Here's how the part is built. I have some questions about the finished solid (model axes, mm). Face numbers are marked on the shaded views. A direction names the side the tool comes from. Give positions to 0.01 mm unless a question says otherwise; leave off trailing zeros. Write each loop counter-clockwise with the first axis right and the second up, starting at its lowest first coordinate (ties: lowest second). Pieces come first, ordered by that corner, then holes. Notation, with made-up numbers: (54, 64.5) -> (103, 64.5) arc R28 ccw to (103, 83.5) -> close; hole circle Ø7 at (73, 81.25). An arc over 180 degrees is marked (long way). Return JSON: item names as keys, results as strings.
from build123d import *

# Parameters (mm, degrees)
F0_R     = 2.5
F0_W     = 19
F0_H     = 3
F0_W_2   = 13
F0_W_3   = 9.5
F0_R_2   = 1.25
F1_DEPTH = 2.5
F2_DEPTH = 15
F3_DEPTH = 6.5
F4_DEPTH = 2.5
F5_DEPTH = 5


# Not quite as in the source:
# - a feature names something its author has since deleted; it is built from what else it names


with BuildPart() as f1:
    # F0 (on Top) → F1 (new body)
    with BuildSketch(Plane.XY):
        Polygon((27.0149873525, -30.0875452161), (27.0149873525, 34.3124547839), (21.4149873525, 39.9124547839), (-12.9189450768, 39.9124547839), (-15.2438546447, 37.5875452161), (-27.5850126475, 37.5875452161), (-27.5850126475, -30.0875452161), (-17.9850126475, -30.0875452161), (-4.9850126475, -30.0875452161), (14.0149873525, -30.0875452161), (23.5149873525, -30.0875452161), align=None)
        with Locations((-24.5850126475, -15.0875452161)):
            Circle(F0_R, mode=Mode.SUBTRACT)
        with Locations((24.0149873525, -16.0875452161)):
            Circle(F0_R, mode=Mode.SUBTRACT)
        with Locations((-8.6850126475, 33.8492766023)):
            Circle(F0_R, mode=Mode.SUBTRACT)
        with Locations((19.3149873525, 33.8492766023)):
            Circle(F0_R, mode=Mode.SUBTRACT)
        Polygon((21.4149873525, 39.9124547839), (27.0149873525, 34.3124547839), (27.0149873525, -30.0875452161), (29.5149873525, -30.0875452161), (29.5149873525, 34.3124547839), (21.5734839439, 42.4124547839), (-13.0739709929, 42.4124547839), (-15.4701419023, 40.0875452161), (-30.0850126475, 40.0875452161), (-30.0850126475, 10), (-30.0850126475, 5), (-30.0850126475, 0), (-30.0850126475, -5), (-30.0850126475, -30.0875452161), (-27.5850126475, -30.0875452161), (-27.5850126475, 37.5875452161), (-15.2438546447, 37.5875452161), (-12.9189450768, 39.9124547839), align=None)
        with Locations((4.5149873525, -31.5875452161)):
            Rectangle(F0_W, F0_H)
        with Locations((-11.4850126475, -31.5875452161)):
            Rectangle(F0_W_2, F0_H)
        Polygon((-17.9850126475, -33.0875452161), (-17.9850126475, -30.0875452161), (-27.5850126475, -30.0875452161), (-30.0850126475, -30.0875452161), (-30.0850126475, -33.0875452161), align=None)
        with Locations((18.7649873525, -31.5875452161)):
            Rectangle(F0_W_3, F0_H)
        with Locations((19.3149873525, 33.8492766023)):
            Circle(F0_R)
        with Locations((19.3149873525, 33.8492766023)):
            Circle(F0_R_2, mode=Mode.SUBTRACT)
        with Locations((-24.5850126475, -15.0875452161)):
            Circle(F0_R)
        with Locations((-24.5850126475, -15.0875452161)):
            Circle(F0_R_2, mode=Mode.SUBTRACT)
        with Locations((24.0149873525, -16.0875452161)):
            Circle(F0_R)
        with Locations((24.0149873525, -16.0875452161)):
            Circle(F0_R_2, mode=Mode.SUBTRACT)
        with Locations((-8.6850126475, 33.8492766023)):
            Circle(F0_R)
        with Locations((-8.6850126475, 33.8492766023)):
            Circle(F0_R_2, mode=Mode.SUBTRACT)
        Polygon((29.5149873525, -30.0875452161), (27.0149873525, -30.0875452161), (23.5149873525, -30.0875452161), (23.5149873525, -33.0875452161), (29.5149873525, -33.0875452161), align=None)
        with Locations((-24.5850126475, -15.0875452161)):
            Circle(F0_R_2)
        with Locations((24.0149873525, -16.0875452161)):
            Circle(F0_R_2)
        with Locations((-8.6850126475, 33.8492766023)):
            Circle(F0_R_2)
        with Locations((19.3149873525, 33.8492766023)):
            Circle(F0_R_2)
    extrude(amount=-F1_DEPTH)

    # F0 (on Top) → F2 (join)
    with BuildSketch(Plane.XY):
        Polygon((21.4149873525, 39.9124547839), (27.0149873525, 34.3124547839), (27.0149873525, -30.0875452161), (29.5149873525, -30.0875452161), (29.5149873525, 34.3124547839), (21.5734839439, 42.4124547839), (-13.0739709929, 42.4124547839), (-15.4701419023, 40.0875452161), (-30.0850126475, 40.0875452161), (-30.0850126475, 10), (-30.0850126475, 5), (-30.0850126475, 0), (-30.0850126475, -5), (-30.0850126475, -30.0875452161), (-27.5850126475, -30.0875452161), (-27.5850126475, 37.5875452161), (-15.2438546447, 37.5875452161), (-12.9189450768, 39.9124547839), align=None)
        Polygon((-17.9850126475, -33.0875452161), (-17.9850126475, -30.0875452161), (-27.5850126475, -30.0875452161), (-30.0850126475, -30.0875452161), (-30.0850126475, -33.0875452161), align=None)
        with Locations((4.5149873525, -31.5875452161)):
            Rectangle(F0_W, F0_H)
        Polygon((29.5149873525, -30.0875452161), (27.0149873525, -30.0875452161), (23.5149873525, -30.0875452161), (23.5149873525, -33.0875452161), (29.5149873525, -33.0875452161), align=None)
    extrude(amount=F2_DEPTH)

    # F0 (on Top) → F3 (join)
    with BuildSketch(Plane.XY):
        with Locations((-11.4850126475, -31.5875452161)):
            Rectangle(F0_W_2, F0_H)
        with Locations((18.7649873525, -31.5875452161)):
            Rectangle(F0_W_3, F0_H)
    extrude(amount=F3_DEPTH)

    # F0 (on Top) → F4 (join)
    with BuildSketch(Plane.XY):
        with BuildLine():
            Line((-35.0850126475, -5), (-30.0850126475, -5))
            Line((-30.0850126475, -5), (-30.0850126475, 0))
            Line((-30.0850126475, 0), (-30.0850126475, 5))
            Line((-30.0850126475, 5), (-35.0850126475, 5))
            ThreePointArc((-35.0850126475, 5), (-38.6205465534, 3.5355339059), (-40.0850126475, 0))
            ThreePointArc((-40.0850126475, 0), (-38.6205465534, -3.5355339059), (-35.0850126475, -5))
        make_face()
        with Locations((-35.0850126475, 0)):
            Circle(F0_R, mode=Mode.SUBTRACT)
    extrude(amount=-F4_DEPTH)

    # F0 (on Top) → F5 (join)
    with BuildSketch(Plane.XY):
        with Locations((-24.5850126475, -15.0875452161)):
            Circle(F0_R)
        with Locations((-24.5850126475, -15.0875452161)):
            Circle(F0_R_2, mode=Mode.SUBTRACT)
        with Locations((-8.6850126475, 33.8492766023)):
            Circle(F0_R)
        with Locations((-8.6850126475, 33.8492766023)):
            Circle(F0_R_2, mode=Mode.SUBTRACT)
        with Locations((19.3149873525, 33.8492766023)):
            Circle(F0_R)
        with Locations((19.3149873525, 33.8492766023)):
            Circle(F0_R_2, mode=Mode.SUBTRACT)
        with Locations((24.0149873525, -16.0875452161)):
            Circle(F0_R)
        with Locations((24.0149873525, -16.0875452161)):
            Circle(F0_R_2, mode=Mode.SUBTRACT)
    extrude(amount=F5_DEPTH)


solid = f1.part
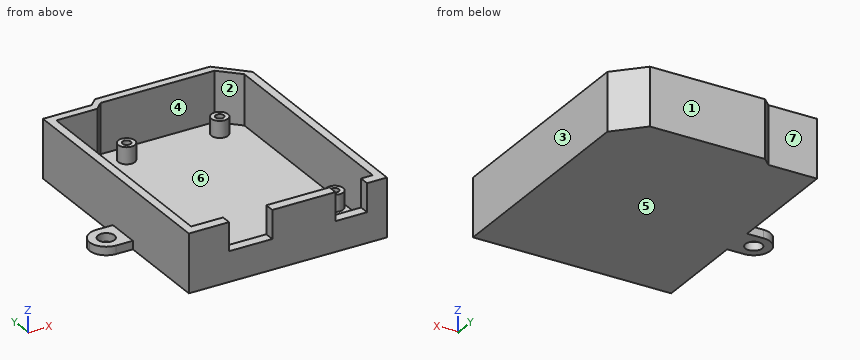
1. Suppose I cut it at A-A, the plane z = 3.25. Count the separate pieces of the cut face and the enclosed holes in it, and give its area (3 significant figures).
Taken from the geometry:
{"separate pieces": "5", "enclosed holes": "5", "area": "715 mm²"}
2. If we mould it in two halves opening along Y, with no side actions, what happens to the marked faces 1, 2, 3 and 4? For each: released by +Y, released by -Y, zero draft, split by the parting line, or undercut.
Taken from the geometry:
{"face 1": "released by +Y", "face 2": "undercut", "face 3": "zero draft", "face 4": "undercut"}
3. Suppose I cut it at B-B, the plane y = 19. List the corners of the cut face in (x, z) for me, and give its area (3 significant figures).
Taken from the geometry:
{"outline": "(-30.09, -2.5) -> (29.51, -2.5) -> (29.51, 15) -> (27.01, 15) -> (27.01, 0) -> (-27.59, 0) -> (-27.59, 15) -> (-30.09, 15) -> close", "area": "224 mm²"}
4. If I drill on line 1 (X direction, y = -18, z = 7.75); line 2 (Y direction, x = -16.5, z = 2); line 3 (Y direction, x = 6, z = 12), over which ranges is the centre line in solid material (lowest first)? Write a range as [from, to].
Taken from the geometry:
{"line 1": "x = [-30.09, -27.59], [27.01, 29.51]", "line 2": "y = [-33.09, -30.09], [37.59, 40.09]", "line 3": "y = [-33.09, -30.09], [39.91, 42.41]"}
5. For pin 1 Ø2 at (x, y) = (19.5, 33.5) entering from +Z; pin 2 Ø5 at (y, z) = (1, 9) entering from -X (3 decimals); pin 3 Ø5 at (x, y) = (14.5, 31.5) entering from +Z, each with a flat end and sliding along its axis, tell me the tip position at first contact or that it passes through.
Taken from the geometry:
{"pin 1": "stops at z = 5", "pin 2": "stops at x = -30.085", "pin 3": "stops at z = 0"}
6. Which directions (+Z, -Z, +X, -X, +Y, -Y) give clear straight access to the entire face, cutting with the end or side of a thin tool? Please do the marked faces 5, 6 and 7.
Taken from the geometry:
{"face 5": "-Z, +X, -X, +Y, -Y", "face 6": "+Z", "face 7": "+Z, -Z, -X, +Y"}
7. Suppose I cut it at C-C, the plane x = -4. List the corners of the cut face in (y, z) for me, and give its area (3 significant figures).
Taken from the geometry:
{"outline": "(-33.09, -2.5) -> (42.41, -2.5) -> (42.41, 15) -> (39.91, 15) -> (39.91, 0) -> (-30.09, 0) -> (-30.09, 15) -> (-33.09, 15) -> close", "area": "271 mm²"}
